Autodesk Inventor part; units mm, degrees
ref_plane "YZ Plane" through (0, 0, 0) normal (1, 0, 0) x (0, 1, 0)
ref_plane "XZ Plane" through (0, 0, 0) normal (0, 1, 0) x (-1, 0, 0)
ref_plane "XY Plane" through (0, 0, 0) normal (0, 0, 1) x (1, 0, 0)
sketch "Boceto1" plane through (0, 0, 0) normal (0, 0, 1) x (1, 0, 0)
  line L0 (-22.25, 73.85) -> (22.25, 73.85)
  line L1 (23.85, 72.25) -> (23.85, -72.25)
  line L2 (22.25, -73.85) -> (-22.25, -73.85)
  line L3 (-23.85, -72.25) -> (-23.85, 72.25)
  line L4 (23.65, -75.25) -> (-23.65, -75.25)
  line L5 (25.25, 73.65) -> (25.25, -73.65)
  line L6 (-23.65, 75.25) -> (23.65, 75.25)
  line L7 (-25.25, -73.65) -> (-25.25, 73.65)
  line L8 (-22.25, 72.25) -> (22.25, 72.25)
  line L9 (-22.25, -72.25) -> (-22.25, 72.25)
  line L10 (22.25, 72.25) -> (22.25, -72.25)
  line L11 (22.25, -72.25) -> (-22.25, -72.25)
  line L12 (25.45, 75.45) -> (-25.45, 75.45)
  line L13 (-25.45, 75.45) -> (-25.45, -75.45)
  line L14 (-25.45, -75.45) -> (25.45, -75.45)
  line L15 (25.45, -75.45) -> (25.45, 75.45)
  arc A0 (23.85, 72.25) -> (22.25, 73.85) centre (22.25, 72.25) ccw
  arc A1 (22.25, -73.85) -> (23.85, -72.25) centre (22.25, -72.25) ccw
  arc A2 (-23.85, -72.25) -> (-22.25, -73.85) centre (-22.25, -72.25) ccw
  arc A3 (-22.25, 73.85) -> (-23.85, 72.25) centre (-22.25, 72.25) ccw
  arc A4 (23.65, -75.25) -> (25.25, -73.65) centre (23.65, -73.65) ccw
  arc A5 (25.25, 73.65) -> (23.65, 75.25) centre (23.65, 73.65) ccw
  arc A6 (-23.65, 75.25) -> (-25.25, 73.65) centre (-23.65, 73.65) ccw
  arc A7 (-25.25, -73.65) -> (-23.65, -75.25) centre (-23.65, -73.65) ccw
  line L16 (-22.25, -74.05) -> (22.25, -74.05)
  arc A8 (22.25, -74.05) -> (24.05, -72.25) centre (22.25, -72.25) ccw
  line L17 (24.05, -72.25) -> (24.05, 72.25)
  arc A9 (24.05, 72.25) -> (22.25, 74.05) centre (22.25, 72.25) ccw
  line L18 (22.25, 74.05) -> (-22.25, 74.05)
  arc A10 (-22.25, 74.05) -> (-24.05, 72.25) centre (-22.25, 72.25) ccw
  line L19 (-24.05, 72.25) -> (-24.05, -72.25)
  arc A11 (-24.05, -72.25) -> (-22.25, -74.05) centre (-22.25, -72.25) ccw
  point P0 (0, 0)
  dimension "d0" = 1.6
  dimension "d10" = 0.2
extrude "Extrusión1" add sketch "Boceto1" along normal blind 9 contours L4 A7 L7 A6 L6 A5 L5 A4 | L15 L14 L13 L12
sketch "Boceto2" plane through (0, 0, 9) normal (0, 0, 1) x (1, 0, 0)
  line L0 (-25.45, 75.45) -> (-25.45, -75.45) construction
  line L1 (-25.45, -75.45) -> (25.45, -75.45) construction
  line L2 (25.45, -75.45) -> (25.45, 75.45) construction
  line L3 (25.45, 75.45) -> (-25.45, 75.45) construction
  line L4 (-22.45, 72.45) -> (-22.45, -72.45)
  line L5 (-22.45, -72.45) -> (22.45, -72.45)
  line L6 (22.45, -72.45) -> (22.45, 72.45)
  line L7 (22.45, 72.45) -> (-22.45, 72.45)
  line L8 (-25.45, 75.45) -> (-25.45, -75.45)
  line L9 (-25.45, -75.45) -> (25.45, -75.45)
  line L10 (25.45, -75.45) -> (25.45, 75.45)
  line L11 (25.45, 75.45) -> (-25.45, 75.45)
  point P0 (0, 0)
  dimension "d3" = 3
  dimension "d4" = 3
extrude "Extrusión2" add sketch "Boceto2" along normal blind 4
sketch "Boceto3" plane through (0, 0, 13) normal (0, 0, 1) x (1, 0, 0)
  line L0 (-25.45, -75.45) -> (25.45, -75.45)
  line L1 (25.45, -75.45) -> (25.45, 75.45)
  line L2 (25.45, 75.45) -> (-25.45, 75.45)
  line L3 (-25.45, 75.45) -> (-25.45, -75.45)
  line L4 (-22.45, 72.45) -> (22.45, 72.45)
  line L5 (22.45, 72.45) -> (22.45, -72.45)
  line L6 (22.45, -72.45) -> (-22.45, -72.45)
  line L7 (-22.45, -72.45) -> (-22.45, 72.45)
  point P0 (0, 0)
extrude "Extrusión3" add sketch "Boceto3" along normal blind 2 contours L3 L2 L1 L0 | L4 L5 L6 L7
fillet "Empalme1" radius 1.6 11 edges at (25.45, -75.45, 12) (25.45, -75.45, 4.5) (-25.45, -75.45, 12) (-25.45, -75.45, 4.5) (-25.45, 75.45, 7.5) (25.45, 75.45, 12) (25.45, 75.45, 4.5) (25.45, 0, 15) (0, 75.45, 15) (-25.45, 0, 15) (0, -75.45, 15)
sketch "Boceto4" plane through (0, 0, 13) normal (0, 0, -1) x (-1, 0, 0)
  line L0 (22.45, -72.45) -> (22.45, 72.45)
  line L1 (22.45, 72.45) -> (-22.45, 72.45)
  line L2 (-22.45, 72.45) -> (-22.45, -72.45)
  line L3 (-22.45, -72.45) -> (22.45, -72.45)
  line L4 (-22.45, -72.45) -> (22.45, -72.45)
  line L5 (-22.45, -72.45) -> (-13.25, -72.45)
  line L6 (-13.25, -72.45) -> (-13.25, -61.35)
  line L7 (-13.25, -61.35) -> (-22.45, -61.35)
  line L8 (-22.45, -61.35) -> (-22.45, -72.45)
  point P0 (0, 0)
  dimension "d11" = 9.2
  dimension "d12" = 11.1
extrude "Extrusión4" cut sketch "Boceto4" against normal blind 9 contours L3 L2 L7 L6
sketch "Boceto5" plane through (0, 0, 13) normal (0, 0, -1) x (-1, 0, 0)
  line L0 (-22.45, -61.35) -> (-13.25, -61.35)
  line L1 (-13.25, -61.35) -> (-13.25, -72.45)
  line L2 (-13.25, -72.45) -> (22.45, -72.45)
  line L3 (22.45, -72.45) -> (22.45, 72.45)
  line L4 (22.45, 72.45) -> (-22.45, 72.45)
  line L5 (-22.45, 72.45) -> (-22.45, -61.35)
  line L6 (-22.45, 72.45) -> (-12.65, 72.45)
  line L7 (-12.65, 72.45) -> (-12.65, 58.15)
  line L8 (-12.65, 58.15) -> (-22.45, 58.15)
  line L9 (-22.45, 58.15) -> (-22.45, 72.45)
  point P0 (0, 0)
  dimension "d15" = 9.8
  dimension "d16" = 14.3
extrude "Extrusión5" cut sketch "Boceto5" against normal blind 9 contours L5 L4 L7 L8
properties part number "Tapa bateria"
The model under review builds one solid part; all positions refer to its coordinate system, in mm. A direction names the side the tool comes from. Round coordinates to 2 decimals unless told otherwise and drop trailing zeros. Order: outer loops, then holes, each group sorted by start corner. A loop starts at its lowest first (then second) coordinate and runs counter-clockwise, first axis right, second up. Notation, with made-up numbers: (-27.75, 5.5) - (13.25, 5.5) arc R24 ccw to (13.25, 32.5) - close; hole circle Ø9 at (15, 28.5). An arc over 180 degrees is marked (long way). Answer in a Markdown table with one row per item.
(1) Take a section at A-A on x = 18.5. Write out the cut boundary in (y, z), plus the area to 3 significant figures.
Result set:
| item | result |
|---|---|
| outline | (-75.45, 0) - (-74.05, 0) - (-74.05, 9) - (-72.45, 9) - (-72.45, 15) - (-73.85, 15) arc R1.6 ccw to (-75.45, 13.4) - close; (-61.35, 13) - (58.15, 13) - (58.15, 15) - (-61.35, 15) - close; (72.45, 9) - (74.05, 9) - (74.05, 0) - (75.45, 0) - (75.45, 13.4) arc R1.6 ccw to (73.85, 15) - (72.45, 15) - close |
| area | 299 mm2 |
(2) Machinability: for faces 1 (the face through (0, -72.45, 11)), 2 (the face through (0, 1, 15)), which of the approach directions +Z, -Z, +X, -X, +Y, -Y give a long, thin tool a straight path to every point of the face, cutting with its end or side? Answer none if there is none.
Result set:
| item | result |
|---|---|
| face 1 | -Z |
| face 2 | +Z, +X, -X, +Y, -Y |
(3) For line 1 (Y direction, x = -10.5, z = 11.5); line 2 (X direction, y = 25.5, z = 7); line 3 (Y direction, x = 12, z = 6), list the stretches that pass through material, from the lowest coordinate up. Write a range as from..to.
Result set:
| item | result |
|---|---|
| line 1 | y = -75.45..-72.45, 72.45..75.45 |
| line 2 | x = -25.45..-24.05, 24.05..25.45 |
| line 3 | y = -75.45..-74.05, 74.05..75.45 |
(4) Take a section at C-C on y = -59.5. Write out the cut boundary in (x, z), plus the area to 3 significant figures.
Result set:
| item | result |
|---|---|
| outline | (-25.45, 0) - (-24.05, 0) - (-24.05, 9) - (-22.45, 9) - (-22.45, 13) - (22.45, 13) - (22.45, 9) - (24.05, 9) - (24.05, 0) - (25.45, 0) - (25.45, 13.4) arc R1.6 ccw to (23.85, 15) - (-23.85, 15) arc R1.6 ccw to (-25.45, 13.4) - close |
| area | 150 mm2 |
(5) Clearance check with flat-ended pins moving along their axes: P1, Ø0.6, axis at x = 15.5, z = 14, coming from the +Y side; P2, Ø8, axis at x = 15.5, y = 52, coming from the -Z side; P3, Ø0.6, axis at x = 16.5, z = 14, coming from the -Y side. State where each tip first meets the part, or that it passes through.
Result set:
| item | result |
|---|---|
| P1 | stops at y = 75.42 |
| P2 | stops at z = 13 |
| P3 | stops at y = -75.42 |
(6) Take a section at D-D on x = 9. Write out the cut boundary in (y, z), plus the area to 3 significant figures.
Result set:
| item | result |
|---|---|
| outline | (-75.45, 0) - (-74.05, 0) - (-74.05, 9) - (-72.45, 9) - (-72.45, 13) - (72.45, 13) - (72.45, 9) - (74.05, 9) - (74.05, 0) - (75.45, 0) - (75.45, 13.4) arc R1.6 ccw to (73.85, 15) - (-73.85, 15) arc R1.6 ccw to (-75.45, 13.4) - close |
| area | 350 mm2 |
(7) Take a section at B-B on z = 6. Write out the cut boundary in (x, y), plus the area to 3 significant figures.
Result set:
| item | result |
|---|---|
| outline | (-25.45, -73.85) arc R1.6 ccw to (-23.85, -75.45) - (23.85, -75.45) arc R1.6 ccw to (25.45, -73.85) - (25.45, 73.85) arc R1.6 ccw to (23.85, 75.45) - (-23.85, 75.45) arc R1.6 ccw to (-25.45, 73.85) - close; hole (-24.05, -72.25) arc R1.8 ccw to (-22.25, -74.05) - (22.25, -74.05) arc R1.8 ccw to (24.05, -72.25) - (24.05, 72.25) arc R1.8 ccw to (22.25, 74.05) - (-22.25, 74.05) arc R1.8 ccw to (-24.05, 72.25) - close |
| area | 558 mm2 |
(8) Mouldability with a two-part tool opening along X and no side actions: class faces 3 (the face through (-25.45, 1, 7)), 4 (the face through (-22.45, 1, 11)), 5 (the face through (25.45, -1, 7)), 6 (the face through (0, -75.45, 7)) as released by +X, released by -X, zero draft, split by the parting line, or undercut.
Result set:
| item | result |
|---|---|
| face 3 | released by -X |
| face 4 | undercut |
| face 5 | released by +X |
| face 6 | zero draft |
